from build123d import *

# Parameters (mm, degrees)
SCHIZZO1_W                   = 61
SCHIZZO1_H                   = 90
ESTRUSIONE_ESTRUSIONE1_DEPTH = 22
SCHIZZO2_W                   = 57.432150226
SCHIZZO2_H                   = 87.001178066
TAGLIO_ESTRUSIONE1_DEPTH     = 20
SCHIZZO3_R                   = 4.288113478
ESTRUSIONE_ESTRUSIONE3_DEPTH = 18
SCHIZZO4_W                   = 18
SCHIZZO4_H                   = 14
TAGLIO_ESTRUSIONE2_DEPTH     = 4
SCHIZZO5_W                   = 28.293055574
SCHIZZO5_H                   = 7.859182103
TAGLIO_ESTRUSIONE4_DEPTH     = 4


with BuildPart() as part:
    # Schizzo1 → Estrusione-Estrusione1 (new body)
    with BuildSketch(Plane.XY):
        with Locations((9.416083916, -18.723776224)):
            Rectangle(SCHIZZO1_W, SCHIZZO1_H)
    extrude(amount=ESTRUSIONE_ESTRUSIONE1_DEPTH)

    # Schizzo2 → Taglio-Estrusione1 (cut)
    with BuildSketch(Plane.XY.offset(22)):
        with Locations((9.321311391, -18.723776224)):
            Rectangle(SCHIZZO2_W, SCHIZZO2_H)
    extrude(amount=-TAGLIO_ESTRUSIONE1_DEPTH, mode=Mode.SUBTRACT)

    # Schizzo3 → Estrusione-Estrusione3 (add)
    with BuildSketch(Plane.XY.offset(2)):
        with Locations(Location((9.233810508, 0, 0), (0, 0, 180))):
            Circle(SCHIZZO3_R)
    extrude(amount=ESTRUSIONE_ESTRUSIONE3_DEPTH)

    # Schizzo4 → Taglio-Estrusione2 (cut)
    with BuildSketch(Plane(origin=(0, -63.723776224, 0), x_dir=(-1, 0, 0), z_dir=(0, -1, 0))):
        with Locations((-14.296265354, -18.438108628)):
            Rectangle(SCHIZZO4_W, SCHIZZO4_H)
    extrude(amount=-TAGLIO_ESTRUSIONE2_DEPTH, mode=Mode.SUBTRACT)

    # Schizzo5 → Taglio-Estrusione4 (cut)
    with BuildSketch(Plane(origin=(0, 26.276223776, 0), x_dir=(1, 0, 0), z_dir=(0, 1, 0))):
        with Locations((18.59196137, -21.617439903)):
            Rectangle(SCHIZZO5_W, SCHIZZO5_H)
    extrude(amount=-TAGLIO_ESTRUSIONE4_DEPTH, mode=Mode.SUBTRACT)


solid = part.part
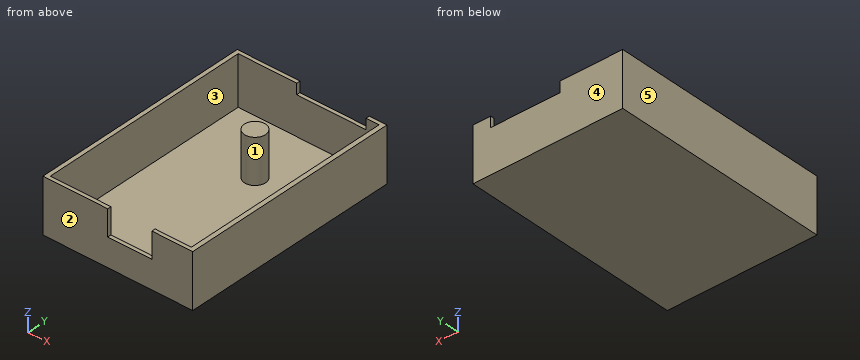
Could you check a few things on this model? Use its own coordinates, in mm. Face numbers are marked on the shaded views. A direction names the side the tool comes from. Give positions to 0.01 mm unless a question says otherwise; leave off trailing zeros. Order: outer loops, then holes, each group sorted by start corner. A loop starts at its lowest first (then second) coordinate and runs counter-clockwise, first axis right, second up.
1. Suppose I cut it at C-C (x = -2.5). List the corners of the cut face in (y, z) for me, plus the area to 3 significant figures.
2. For the marked faces 1 and 2, which set-ups out of +Z, -Z, +X, -X, +Y, -Y let a thin tool reach every point of the face, with its end or its side?
3. We'd pull the mould along Y, two halves only. Please class the marked faces 3, 4 and 5: pulls with the +Y half, pulls with the -Y half, needs draft (parallel to the pull), parting line crosses it, or undercut.
4. Suppose I cut it at A-A (z = 8). List the corners of the cut face in (x, y) for me, plus the area to 3 significant figures.
5. I need wall thicknesses on L1, parallel to X at y = 7.5, z = 20.25; L2, parallel to Y at x = 30, z = 3.5; L3, parallel to Z at x = -16, y = -25.5. Which ranges of each line are inside material? Lowest first, please.
6. Will these pins go through, and if not, where does the flat tip stop? P1, Ø1.6, axis at x = 14.5, y = 25.5, coming from the +Z side; P2, Ø2.5, axis at x = 8, y = 1.5, coming from the +Z side.
7. Suppose I cut it at D-D (y = -37). List the corners of the cut face in (x, z) for me.
8. Suppose I cut it at B-B (y = 0). List the corners of the cut face in (x, z) for me.
Solved:
1. outline: (-63.72, 0) - (26.28, 0) - (26.28, 22) - (24.78, 22) - (24.78, 2) - (-62.22, 2) - (-62.22, 22) - (-63.72, 22) - close
1. area: 240 mm2
2. face 1: +Z
2. face 2: +Z, -Z, +X, -X, -Y
3. face 3: undercut
3. face 4: pulls with the +Y half
3. face 5: needs draft
4. outline: (-21.08, -63.72) - (39.92, -63.72) - (39.92, 26.28) - (-21.08, 26.28) - close; circle Ø8.58 at (9.23, 0); hole (-19.39, -62.22) - (38.04, -62.22) - (38.04, 24.78) - (-19.39, 24.78) - close
4. area: 551 mm2
5. L1: x = -21.08 to -19.39, 38.04 to 39.92
5. L2: y = -63.72 to -62.22, 24.78 to 26.28
5. L3: z = 0 to 2
6. P1: stops at z = 17.69
6. P2: stops at z = 20
7. outline: (-21.08, 0) - (39.92, 0) - (39.92, 22) - (38.04, 22) - (38.04, 2) - (-19.39, 2) - (-19.39, 22) - (-21.08, 22) - close
8. outline: (-21.08, 0) - (39.92, 0) - (39.92, 22) - (38.04, 22) - (38.04, 2) - (13.52, 2) - (13.52, 20) - (4.95, 20) - (4.95, 2) - (-19.39, 2) - (-19.39, 22) - (-21.08, 22) - close
